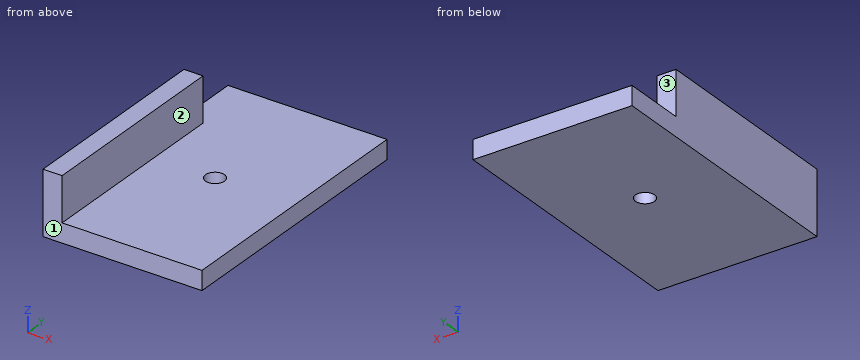
from build123d import *

# Parameters (mm, degrees)
SKETCH_1_W          = 25
SKETCH_1_H          = 42
SKETCH_1_R          = 1.5
EXTRUDE_1_DEPTH     = 3
SKETCH_2_W          = 3
SKETCH_2_H          = 42
EXTRUDE_2_DEPTH     = 7
SKETCH_4_W          = 7
SKETCH_4_H          = 10
CUT_EXTRUDE_1_DEPTH = 10


with BuildPart() as part:
    # 草图1 → 凸台-拉伸1 (new body)
    with BuildSketch(Plane.XY):
        Rectangle(SKETCH_1_W, SKETCH_1_H)
        Circle(SKETCH_1_R, mode=Mode.SUBTRACT)
    extrude(amount=EXTRUDE_1_DEPTH)

    # 草图2 → 凸台-拉伸2 (add)
    with BuildSketch(Plane.XY.offset(3)):
        with Locations((-11, 0)):
            Rectangle(SKETCH_2_W, SKETCH_2_H)
    extrude(amount=EXTRUDE_2_DEPTH)

    # 草图4 → 切除-拉伸1 (cut)
    with BuildSketch(Plane(origin=(-9.5, 0, 0), x_dir=(0, 0, -1), z_dir=(1, 0, 0))):
        with Locations((-6.5, 16)):
            Rectangle(SKETCH_4_W, SKETCH_4_H)
    extrude(amount=-CUT_EXTRUDE_1_DEPTH, mode=Mode.SUBTRACT)


solid = part.part
Could you check a few things on this model? Use its own coordinates, in mm. Face numbers are marked on the shaded views. A direction names the side the tool comes from. Round coordinates to 2 decimals unless told otherwise and drop trailing zeros. Order: outer loops, then holes, each group sorted by start corner. A loop starts at its lowest first (then second) coordinate and runs counter-clockwise, first axis right, second up.
Q1. Imagine slicing it at A-A, the plane x = 0. List the corners of the cut face in (y, z) for me, then the cut area to 3 significant figures.
Geometry says:
outline: (-21, 0) - (-1.5, 0) - (-1.5, 3) - (-21, 3) - close; (1.5, 0) - (21, 0) - (21, 3) - (1.5, 3) - close
area: 117 mm2
Q2. Please list where these lines run through material, in increasing order: probe 1 along Y at (x, z) = (0, 0.8); probe 2 along X at (y, z) = (-16.5, 5); probe 3 along Y at (x, z) = (0.5, 0.5).
Geometry says:
probe 1: y = -21 to -1.5, 1.5 to 21
probe 2: x = -12.5 to -9.5
probe 3: y = -21 to -1.41, 1.41 to 21
Q3. Imagine slicing it at B-B, the plane y = 0. List the corners of the cut face in (x, z) for me, then the cut area to 3 significant figures.
Geometry says:
outline: (-12.5, 0) - (-1.5, 0) - (-1.5, 3) - (-9.5, 3) - (-9.5, 10) - (-12.5, 10) - close; (1.5, 0) - (12.5, 0) - (12.5, 3) - (1.5, 3) - close
area: 87.0 mm2
Q4. Imagine slicing it at D-D, the plane z = 6.25. List the corners of the cut face in (x, y) for me.
Geometry says:
outline: (-12.5, -21) - (-9.5, -21) - (-9.5, 11) - (-12.5, 11) - close
Q5. Imagine slicing it at C-C, the plane y = -17. List the corners of the cut face in (x, z) for me.
Geometry says:
outline: (-12.5, 0) - (12.5, 0) - (12.5, 3) - (-9.5, 3) - (-9.5, 10) - (-12.5, 10) - close
Q6. I'm going to push flat-ended pins straight in: P1, Ø3.5, axis at x = -10.5, z = 8, coming from the +Y side; P2, Ø5.5, axis at y = -3, z = 7, coming from the +X side; P3, Ø4, axis at x = 9.5, y = -12.5, coming from the +Z side. Where does each tip first touch, or does it pass through?
Geometry says:
P1: stops at y = 11
P2: stops at x = -9.5
P3: stops at z = 3
Q7. Which directions (+Z, -Z, +X, -X, +Y, -Y) give clear straight access to the entire face, cutting with the end or side of a thin tool? Please do the marked faces 1, 2 and 3.
Geometry says:
face 1: +Z, -Z, +X, -X, -Y
face 2: +Z, +X, +Y, -Y
face 3: +Z, +X, -X, +Y
